Can you work these out from the model? Positions are in its coordinate system, mm. A direction names the side the tool comes from. Round coordinates to 2 decimals unless told otherwise and drop trailing zeros. Loops run counter-clockwise (first coordinate to the right, second up) from the corner with the lowest first, then second, coordinate; pieces in that order, holes last. Notation, with made-up numbers: M -4.75,-1.75 L 54.25,-1.75 A14 cw 54.25,7.25 Z; hole C -30,2.25 d10. An arc over 180 degrees is marked long. Answer as CSV lines item,"result".
from build123d import *

# Parameters (mm, degrees)
SKETCH_1_R           = 6
EXTRUDE_1_DEPTH      = 3
SKETCH_1_3_R         = 4.7
EXTRUDE_2_DEPTH      = 3.6
SKETCH_1_4_R         = 2.5
CUT_EXTRUDE_1_DEPTH  = 3.6
SKETCH_1_7_R         = 17.3
EXTRUDE_4_DEPTH      = 15.3
SKETCH_1_8_R         = 17.3
SKETCH_1_8_R_2       = 16.75
CUT_EXTRUDE_3_DEPTH  = 4.35
SKETCH_1_5_R         = 17.3
EXTRUDE_3_DEPTH      = 3.85
SKETCH_1_6_R         = 17.3
SKETCH_1_6_R_2       = 16.75
CUT_EXTRUDE_2_DEPTH  = 1
SKETCH_5_R           = 3.25
CUT_EXTRUDE_4_DEPTH  = 10.6
SKETCH_5_3_R         = 1.25
SKETCH_5_3_R_2       = 1
CUT_EXTRUDE_5_DEPTH  = 2.5
SKETCH_1_9_R         = 1.25
SKETCH_1_9_R_2       = 1
CUT_EXTRUDE_6_DEPTH  = 3.8
FILLET_1_R           = 0.7
CHAMFER_1_SIZE       = 0.5
CUT_EXTRUDE_START    = -10
SKETCH_1_10_R        = 2.5
CUT_EXTRUDE_7_DEPTH  = 10
CUT_EXTRUDE_8_DEPTH  = 0.3
EXTRUDE_5_DEPTH      = 0.45
EXTRUDE_5_2_DEPTH    = 0.45
EXTRUDE_5_3_DEPTH    = 0.45
EXTRUDE_6_DEPTH      = 0.3
FILLET_2_R           = 0.75
FILLET_3_R           = 0.75
FILLET_4_R           = 0.75
EXTRUDE_7_DEPTH      = 0.3
SKETCH_1_13_R        = 0.5
CUT_EXTRUDE_9_DEPTH  = 2
CUT_EXTRUDE_10_DEPTH = 0.2


with BuildPart() as part:
    # Sketch 1 → Extrude 1 (new body)
    with BuildSketch(Plane.XY):
        Circle(SKETCH_1_R)
    extrude(amount=EXTRUDE_1_DEPTH)

    # Sketch 1_3 → Extrude 2 (add)
    with BuildSketch(Plane.XY):
        Circle(SKETCH_1_3_R)
    extrude(amount=EXTRUDE_2_DEPTH)

    # Sketch 1_4 → Cut-Extrude 1 (cut)
    with BuildSketch(Plane.XY):
        Circle(SKETCH_1_4_R)
    extrude(amount=CUT_EXTRUDE_1_DEPTH, mode=Mode.SUBTRACT)

    # Sketch 1_7 → Extrude 4 (add)
    with BuildSketch(Plane.XY):
        Circle(SKETCH_1_7_R)
    extrude(amount=-EXTRUDE_4_DEPTH)

    # Sketch 1_8 → Cut-Extrude 3 (cut)
    with BuildSketch(Plane.XY):
        Circle(SKETCH_1_8_R)
        Circle(SKETCH_1_8_R_2, mode=Mode.SUBTRACT)
    extrude(amount=-CUT_EXTRUDE_3_DEPTH, mode=Mode.SUBTRACT)

    # Sketch 1_5 → Extrude 3 (add)
    with BuildSketch(Plane.XY):
        Circle(SKETCH_1_5_R)
    extrude(amount=-EXTRUDE_3_DEPTH)

    # Sketch 1_6 → Cut-Extrude 2 (cut)
    with BuildSketch(Plane.XY):
        Circle(SKETCH_1_6_R)
        Circle(SKETCH_1_6_R_2, mode=Mode.SUBTRACT)
    extrude(amount=-CUT_EXTRUDE_2_DEPTH, mode=Mode.SUBTRACT)

    # Sketch 5 → Cut-Extrude 4 (cut)
    with BuildSketch(Plane(origin=(0, 0, -15.3), x_dir=(-1, 0, 0), z_dir=(0, 0, -1))):
        Circle(SKETCH_5_R)
    extrude(amount=-CUT_EXTRUDE_4_DEPTH, mode=Mode.SUBTRACT)

    # Sketch 5_3 → Cut-Extrude 5 (cut)
    with BuildSketch(Plane(origin=(0, 0, -15.3), x_dir=(-1, 0, 0), z_dir=(0, 0, -1))):
        with Locations((-5.25, 5.25)):
            Circle(SKETCH_5_3_R)
        with Locations((0, 6.25)):
            Circle(SKETCH_5_3_R_2)
        with Locations((5.25, 5.25)):
            Circle(SKETCH_5_3_R)
        with Locations((6.25, 0)):
            Circle(SKETCH_5_3_R_2)
        with Locations((5.25, -5.25)):
            Circle(SKETCH_5_3_R)
        with Locations((0, -6.25)):
            Circle(SKETCH_5_3_R_2)
        with Locations((-5.25, -5.25)):
            Circle(SKETCH_5_3_R)
        with Locations((-6.25, 0)):
            Circle(SKETCH_5_3_R_2)
    extrude(amount=-CUT_EXTRUDE_5_DEPTH, mode=Mode.SUBTRACT)

    # Sketch 1_9 → Cut-Extrude 6 (cut)
    with BuildSketch(Plane.XY):
        with Locations((0, 14.75)):
            Circle(SKETCH_1_9_R)
        with Locations((8, 10.25)):
            Circle(SKETCH_1_9_R_2)
        with Locations((8, -10.25)):
            Circle(SKETCH_1_9_R_2)
        with Locations((0, -14.75)):
            Circle(SKETCH_1_9_R)
        with Locations((-8, -10.25)):
            Circle(SKETCH_1_9_R_2)
        with Locations((-8, 10.25)):
            Circle(SKETCH_1_9_R_2)
    extrude(amount=-CUT_EXTRUDE_6_DEPTH, mode=Mode.SUBTRACT)

    # Fillet 1
    fillet_1_edges = [part.edges().sort_by_distance(p)[0] for p in [
        (-17.3, 0, -15.3),
    ]]
    fillet(fillet_1_edges, radius=FILLET_1_R)

    # Chamfer 1
    chamfer_1_edges = [part.edges().sort_by_distance(p)[0] for p in [
        (-6, 0, 3),
    ]]
    chamfer(chamfer_1_edges, length=CHAMFER_1_SIZE)

    # Sketch 1_10 → Cut-Extrude 7 (cut)
    with BuildSketch(Plane.XY.offset(CUT_EXTRUDE_START)):
        with Locations(Location((0, 0, 0), (0, 0, 180))):
            Circle(SKETCH_1_10_R)
    extrude(amount=CUT_EXTRUDE_7_DEPTH, mode=Mode.SUBTRACT)

    # Sketch 1_11 → Cut-Extrude 8 (cut)
    with BuildSketch(Plane.XY):
        with BuildLine():
            Line((-9.5, 6), (-13.5, 6))
            ThreePointArc((-13.5, 6), (-14.560660172, 5.560660172), (-15, 4.5))
            Line((-15, 4.5), (-15, -4.5))
            ThreePointArc((-15, -4.5), (-14.560660172, -5.560660172), (-13.5, -6))
            Line((-13.5, -6), (-9.5, -6))
            ThreePointArc((-9.5, -6), (-8.439339828, -5.560660172), (-8, -4.5))
            Line((-8, -4.5), (-8, 4.5))
            ThreePointArc((-8, 4.5), (-8.439339828, 5.560660172), (-9.5, 6))
        make_face()
    extrude(amount=-CUT_EXTRUDE_8_DEPTH, mode=Mode.SUBTRACT)



with BuildPart() as body_2:
    # Sketch 1_12 → Extrude 5 (new body)
    with BuildSketch(Plane.XY):
        with BuildLine():
            ThreePointArc((-9, 0.75), (-8.25, 0), (-9, -0.75))
            Line((-9, -0.75), (-10.5, -0.75))
            ThreePointArc((-10.5, -0.75), (-11.25, 0), (-10.5, 0.75))
            Line((-10.5, 0.75), (-9, 0.75))
        make_face()
    extrude(amount=EXTRUDE_5_DEPTH)


with BuildPart() as body_3:
    # Sketch 1_12 → Extrude 5 2 (new body)
    with BuildSketch(Plane.XY):
        with BuildLine():
            ThreePointArc((-9, -1.45), (-8.25, -2.2), (-9, -2.95))
            Line((-9, -2.95), (-10.5, -2.95))
            ThreePointArc((-10.5, -2.95), (-11.25, -2.2), (-10.5, -1.45))
            Line((-10.5, -1.45), (-9, -1.45))
        make_face()
    extrude(amount=EXTRUDE_5_2_DEPTH)


with BuildPart() as body_4:
    # Sketch 1_12 → Extrude 5 3 (new body)
    with BuildSketch(Plane.XY):
        with BuildLine():
            ThreePointArc((-9, 2.95), (-8.25, 2.2), (-9, 1.45))
            Line((-9, 1.45), (-10.5, 1.45))
            ThreePointArc((-10.5, 1.45), (-11.25, 2.2), (-10.5, 2.95))
            Line((-10.5, 2.95), (-9, 2.95))
        make_face()
    extrude(amount=EXTRUDE_5_3_DEPTH)


with BuildPart() as part_1:
    add(part.part)

    add(body_2.part)  # Extrude 6 merges body 2

    add(body_3.part)  # Extrude 6 merges body 3

    add(body_4.part)  # Extrude 6 merges body 4
    # Sketch 1_14 → Extrude 6 (add)
    with BuildSketch(Plane.XY):
        with BuildLine():
            Line((-10.5, -0.75), (-9, -0.75))
            ThreePointArc((-9, -0.75), (-8.25, 0), (-9, 0.75))
            Line((-9, 0.75), (-10.5, 0.75))
            ThreePointArc((-10.5, 0.75), (-11.25, 0), (-10.5, -0.75))
        make_face()
        with BuildLine():
            Line((-10.5, -2.95), (-9, -2.95))
            ThreePointArc((-9, -2.95), (-8.25, -2.2), (-9, -1.45))
            Line((-9, -1.45), (-10.5, -1.45))
            ThreePointArc((-10.5, -1.45), (-11.25, -2.2), (-10.5, -2.95))
        make_face()
        with BuildLine():
            Line((-10.5, 1.45), (-9, 1.45))
            ThreePointArc((-9, 1.45), (-8.25, 2.2), (-9, 2.95))
            Line((-9, 2.95), (-10.5, 2.95))
            ThreePointArc((-10.5, 2.95), (-11.25, 2.2), (-10.5, 1.45))
        make_face()
    extrude(amount=-EXTRUDE_6_DEPTH)

    # Fillet 2
    fillet_2_edges = [part_1.edges().sort_by_distance(p)[0] for p in [
        (-11.25, 2.2, 0.45),
        (-9.75, 1.45, 0.45),
        (-8.25, 2.2, 0.45),
        (-9.75, 2.95, 0.45),
    ]]
    fillet(fillet_2_edges, radius=FILLET_2_R - 0.0001)  # a hair under: the kernel refuses the full size

    # Fillet 3
    fillet_3_edges = [part_1.edges().sort_by_distance(p)[0] for p in [
        (-11.25, 0, 0.45),
        (-9.75, -0.75, 0.45),
        (-8.25, 0, 0.45),
        (-9.75, 0.75, 0.45),
    ]]
    fillet(fillet_3_edges, radius=FILLET_3_R - 0.0001)  # a hair under: the kernel refuses the full size

    # Fillet 4
    fillet_4_edges = [part_1.edges().sort_by_distance(p)[0] for p in [
        (-11.25, -2.2, 0.45),
        (-9.75, -2.95, 0.45),
        (-8.25, -2.2, 0.45),
        (-9.75, -1.45, 0.45),
    ]]
    fillet(fillet_4_edges, radius=FILLET_4_R - 0.0001)  # a hair under: the kernel refuses the full size

    # Sketch 1_15 → Extrude 7 (add)
    with BuildSketch(Plane.XY):
        with BuildLine():
            Line((-12.5, -0.75), (-14, -0.75))
            ThreePointArc((-14, -0.75), (-14.75, 0), (-14, 0.75))
            Line((-14, 0.75), (-12.5, 0.75))
            ThreePointArc((-12.5, 0.75), (-11.75, 0), (-12.5, -0.75))
        make_face()
        with BuildLine():
            Line((-12.5, 1.45), (-14, 1.45))
            ThreePointArc((-14, 1.45), (-14.75, 2.2), (-14, 2.95))
            Line((-14, 2.95), (-12.5, 2.95))
            ThreePointArc((-12.5, 2.95), (-11.75, 2.2), (-12.5, 1.45))
        make_face()
        with BuildLine():
            Line((-12.5, -2.95), (-14, -2.95))
            ThreePointArc((-14, -2.95), (-14.75, -2.2), (-14, -1.45))
            Line((-14, -1.45), (-12.5, -1.45))
            ThreePointArc((-12.5, -1.45), (-11.75, -2.2), (-12.5, -2.95))
        make_face()
    extrude(amount=-EXTRUDE_7_DEPTH)

    # Sketch 1_13 → Cut-Extrude 9 (cut)
    with BuildSketch(Plane.XY):
        with Locations((-12.5, 0)):
            Circle(SKETCH_1_13_R)
        with Locations((-12.5, 2.2)):
            Circle(SKETCH_1_13_R)
        with Locations((-12.5, -2.2)):
            Circle(SKETCH_1_13_R)
    extrude(amount=-CUT_EXTRUDE_9_DEPTH, mode=Mode.SUBTRACT)

    # Sketch 1_16 → Cut-Extrude 10 (cut)
    with BuildSketch(Plane.XY):
        with BuildLine():
            Line((-12.5, -0.75), (-14, -0.75))
            ThreePointArc((-14, -0.75), (-14.75, 0), (-14, 0.75))
            Line((-14, 0.75), (-12.5, 0.75))
            ThreePointArc((-12.5, 0.75), (-11.75, 0), (-12.5, -0.75))
        make_face()
        with BuildLine():
            Line((-12.5, 1.45), (-14, 1.45))
            ThreePointArc((-14, 1.45), (-14.75, 2.2), (-14, 2.95))
            Line((-14, 2.95), (-12.5, 2.95))
            ThreePointArc((-12.5, 2.95), (-11.75, 2.2), (-12.5, 1.45))
        make_face()
        with BuildLine():
            Line((-12.5, -2.95), (-14, -2.95))
            ThreePointArc((-14, -2.95), (-14.75, -2.2), (-14, -1.45))
            Line((-14, -1.45), (-12.5, -1.45))
            ThreePointArc((-12.5, -1.45), (-11.75, -2.2), (-12.5, -2.95))
        make_face()
    extrude(amount=-CUT_EXTRUDE_10_DEPTH, mode=Mode.SUBTRACT)


solid = part_1.part
Item 1: If we section it at A-A on z = -9.5: Write out the boundary of the cut face in (x, y).
Output:
outline,"C 0,0 d34.6; hole C 0,0 d6.5"
Item 2: We'd pull the mould along X, two halves only. Please class faces 3 (the face through (6, 0, -12.8)), 4 (the face through (-17, 1, -4.35)): released by +X, released by -X, zero draft, split by the parting line, or undercut.
Output:
face 3,"undercut"
face 4,"zero draft"
Item 3: Will these pins go through, and if not, where does the flat tip stop? pin 1 (0.6 mm diameter, centred on x = 6, y = -0.5, fed in from -Z); pin 2 (1.2 mm diameter, centred on x = -0.5, y = 15, fed in from +Z); pin 3 (0.5 mm diameter, centred on x = -12.5, y = 2, fed in from +Z).
Output:
pin 1,"stops at z = -12.8"
pin 2,"stops at z = -3.8"
pin 3,"stops at z = -2"
Item 4: If I drill on line 1 along Y through (x, z) = (0, -2.1); line 2 along Y through (x, z) = (0, -11.25); line 3 along Y through (x, z) = (-6.25, -13.9), over which ranges is the centre line in solid material (lowest first)? Write a range as from..to.
Output:
line 1,"y = -17.3..-16, -13.5..-2.5, 2.5..13.5, 16..17.3"
line 2,"y = -17.3..-3.25, 3.25..17.3"
line 3,"y = -16.13..-6, -4.5..-1, 1..4.5, 6..16.13"
Item 5: On a 3-axis mill with a long thin cutter (end or side, diameter ignored), from which of +Z, -Z, +X, -X, +Y, -Y can I reach the whole of each face in a straight line? I mean faces 1 (the face through (-4.98, -6.47, -14.07)), 2 (the face through (0, 16, -2)). Say none if no direction works.
Output:
face 1,"-Z"
face 2,"+Z"
